Can you work these out from the model? Positions are in its coordinate system, mm. Face numbers are marked on the shaded views. Give positions to 0.01 mm unless a question says otherwise; leave off trailing zeros. Write each loop counter-clockwise with the first axis right and the second up, starting at its lowest first coordinate (ties: lowest second). Pieces come first, ordered by that corner, then holes.
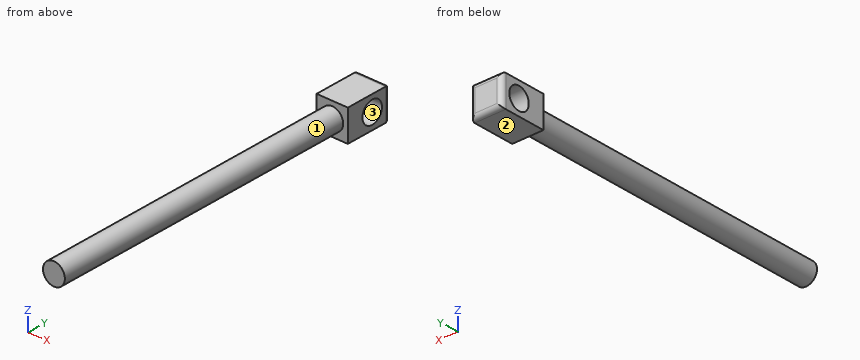
```python
from build123d import *

# Parameters (mm, degrees)
SKETCH1_R           = 17.78
BOSS_EXTRUDE1_DEPTH = 508
SKETCH2_W           = 50.8
SKETCH2_H           = 50.8
BOSS_EXTRUDE2_DEPTH = 76.2
SKETCH4_R           = 17.78
CUT_EXTRUDE1_DEPTH  = 587.954376421
FILLET1_R           = 7.62
SCALE1_SCALE        = 2


with BuildPart() as part:
    # Sketch1 → Boss-Extrude1 (new body)
    with BuildSketch(Plane(origin=(0, 0, 0), x_dir=(1, 0, 0), z_dir=(0, 1, 0))):
        with Locations(Location((0, 0, 0), (0, 0, 270))):
            Circle(SKETCH1_R)
    extrude(amount=BOSS_EXTRUDE1_DEPTH)

    # Sketch2 → Boss-Extrude2 (add)
    with BuildSketch(Plane(origin=(0, 508, 0), x_dir=(1, 0, 0), z_dir=(0, 1, 0))):
        Rectangle(SKETCH2_W, SKETCH2_H)
    extrude(amount=BOSS_EXTRUDE2_DEPTH)

    # Sketch4 → Cut-Extrude1 (cut, through all)
    with BuildSketch(Plane.ZY.offset(25.4)):
        with Locations((0, 552.501368348)):
            Circle(SKETCH4_R)
    extrude(amount=-CUT_EXTRUDE1_DEPTH, mode=Mode.SUBTRACT)

    # Fillet1
    fillet1_edges = [part.edges().sort_by_distance(p)[0] for p in [
        (25.4, 584.2, 0),
        (0, 584.2, -25.4),
        (-25.4, 584.2, 0),
        (0, 584.2, 25.4),
    ]]
    fillet(fillet1_edges, radius=FILLET1_R)


with BuildPart() as part_1:
    # Scale1: scaled about (0, 318.169265299, 0)
    add(part.part.scale(SCALE1_SCALE).moved(Location((0, -318.169265299, 0))))


solid = part_1.part
```
1) If we mould it in two halves opening along Z, with no side actions, what happens to the marked faces 1, 2 and 3? For each: +Z half, -Z half, draft (parallel to the pull), parting line (faces both ways), or undercut.
Values follow:
face 1: parting line
face 2: -Z half
face 3: undercut
2) Suppose I cut it at A-A on z = 0. Write out the boundary of the cut face in (x, y).
Values follow:
outline: (-50.8, 697.83) - (-35.56, 697.83) - (-35.56, -318.17) - (35.56, -318.17) - (35.56, 697.83) - (50.8, 697.83) - (50.8, 751.27) - (-50.8, 751.27) - close; (-50.8, 822.39) - (50.8, 822.39) - (50.8, 834.99) arc R15.24 ccw to (35.56, 850.23) - (-35.56, 850.23) arc R15.24 ccw to (-50.8, 834.99) - close
3) Suppose I cut it at C-C on y = 129. Write out the boundary of the cut face in (x, z), plus the area to 3 significant figures.
Values follow:
outline: circle Ø71.12 at (0, 0)
area: 3,970 mm2
4) For pin 1 Ø12 at (y, z) = (684.5, 34) entering from +X; pin 2 Ø2 at (x, z) = (21.5, -39) entering from -Y; pin 3 Ø12 at (x, y) = (-17, 376) entering from -Z, each with a flat end and sliding along its axis, tell me the tip position at first contact or that it passes through.
Values follow:
pin 1: stops at x = 21.92
pin 2: stops at y = 697.83
pin 3: stops at z = -33.82
5) Please list where these lines run through material, in increasing order: L1, parallel to Y at x = 23.5, z = 0; L2, parallel to Y at x = 9.5, z = -36; L3, parallel to Y at x = -7, z = -24.
Values follow:
L1: y = -318.17 to 751.27, 822.39 to 850.23
L2: y = 697.83 to 850.22
L3: y = -318.17 to 760.59, 813.07 to 850.23
6) Suppose I cut it at B-B on x = -20.5. Write out the boundary of the cut face in (y, z), plus the area to 3 significant figures.
Values follow:
outline: (-318.17, -29.06) - (697.83, -29.06) - (697.83, -50.8) - (834.99, -50.8) arc R15.24 ccw to (850.23, -35.56) - (850.23, 35.56) arc R15.24 ccw to (834.99, 50.8) - (697.83, 50.8) - (697.83, 29.06) - (-318.17, 29.06) - close; hole circle Ø71.12 at (786.83, 0)
area: 70,500 mm2
